Geometry: final body of the model. Coordinates: model frame, mm. A direction names the side the tool comes from. Give positions to 0.01 mm unless a question says otherwise; leave off trailing zeros. Loops run counter-clockwise (first coordinate to the right, second up) from the corner with the lowest first, then second, coordinate; pieces in that order, holes last. Notation, with made-up numbers: (12, -15) -> (63, -15) arc R19 cw to (63, 3) -> close; hole circle Ø9 at (-8, 59.5). An arc over 180 degrees is marked (long way). Answer in a Markdown table with one row per item. Add a question column.
1) Section query D-D (x = 2). Return the cut outline in (y, z), plus the area to 3 significant figures.
2) Section query A-A (z = -4.38). Return the cut outline in (x, y).
3) Section query B-B (y = 2.4). Return the cut outline in (x, z), plus the area to 3 significant figures.
4) Draft query along Z for faces 1 (the flat face through (4.52, 1.48, -21.69)), 2 (the flat face through (5, 3, -12)), 3 (the cylindrical face through (3.79, 1.48, -4.05)). Return one class per face: +Z half, -Z half, draft (parallel to the pull), parting line (faces both ways), or undercut.
5) Section query C-C (z = -21). Return the cut outline in (x, y).
6) Access query for faces 4 (the flat face through (6.006, 1.479, -21.651)), 5 (the flat face through (9.254, 1, -11)). Directions: +Z, -Z, +X, -X, +Y, -Y. A direction counts if a zero-diameter tool reaches every point of the face in a straight line with its end or side. Return the directions, or none.
7) First-contact query: P1, Ø2.5, axis at x = 5.25, z = -14.38, coming from the -Y side. Flat tip, straight axial feed; report the tip coordinate or a pass-through.
8) Line query: line 1 (Z direction, x = 5.25, y = 2.65); line 2 (X direction, y = 2.05, z = -14.38); line 3 (Z direction, x = 5.75, y = 2.4). Output: solid intervals per line, ascending. Write a range as from..to.
```python
from build123d import *

# Parameters (mm, degrees)
BOSS_EXTRUDE3_DEPTH      = 3
M3_CLEARANCE_HOLE1_D     = 3
M3_CLEARANCE_HOLE1_DEPTH = 10
M3_CLEARANCE_HOLE1_TIP   = 0.901290929
SKETCH5_W                = 0.5
SKETCH5_H                = 21.724414851
CUT_EXTRUDE1_DEPTH       = 10
SKETCH6_W                = 8
SKETCH6_H                = 3
CUT_EXTRUDE2_DEPTH       = 1.38


with BuildPart() as part:
    # Sketch1 → Boss-Extrude3 (new body)
    with BuildSketch(Plane(origin=(0, 0, 0), x_dir=(1, 0, 0), z_dir=(0, 1, 0))):
        Polygon((5.303721661, 23.00020151), (5.253721661, 23.00020151), (5.253721661, 0), (9.753721661, 0), (9.753721661, 21.724414851), (9.35, 21.724414851), (6.6889675, 20.339169011), align=None)
        Polygon((3.818475821, 20.339169011), (1.157443322, 21.724414851), (0.753721661, 21.724414851), (0.753721661, 0), (5.253721661, 0), (5.253721661, 23.00020151), (5.203721661, 23.00020151), align=None)
    extrude(amount=BOSS_EXTRUDE3_DEPTH)

    # M3 Clearance Hole1
    with Locations(Plane(origin=(5.253721661, 3, -14.38), x_dir=(0, 0, 1), z_dir=(0, 1, 0))):
        with Locations((0, 0), (10, 0)):
            Hole(M3_CLEARANCE_HOLE1_D / 2, depth=M3_CLEARANCE_HOLE1_DEPTH)
            with Locations((0, 0, -(M3_CLEARANCE_HOLE1_DEPTH + M3_CLEARANCE_HOLE1_TIP / 2))):  # 118° drill point
                Cone(0, M3_CLEARANCE_HOLE1_D / 2, M3_CLEARANCE_HOLE1_TIP, mode=Mode.SUBTRACT)

    # Sketch5 → Cut-Extrude1 (cut)
    with BuildSketch(Plane(origin=(0, 0, 0), x_dir=(-1, 0, 0), z_dir=(0, -1, 0))):
        with Locations((-1.003721661, 10.862207426)):
            Rectangle(SKETCH5_W, SKETCH5_H)
        with Locations((-9.503721661, 10.862207426)):
            Rectangle(SKETCH5_W, SKETCH5_H)
    extrude(amount=-CUT_EXTRUDE1_DEPTH, mode=Mode.SUBTRACT)

    # Sketch6 → Cut-Extrude2 (cut)
    with BuildSketch(Plane.XY):
        with Locations((5.253721661, 1.5)):
            Rectangle(SKETCH6_W, SKETCH6_H)
    extrude(amount=-CUT_EXTRUDE2_DEPTH, mode=Mode.SUBTRACT)


solid = part.part
```
Evaluation:
| question | item | result |
|---|---|---|
| 1 | outline | (0, -21.29) -> (3, -21.29) -> (3, -1.38) -> (0, -1.38) -> close |
| 1 | area | 59.7 mm² |
| 2 | outline | (1.25, 0) -> (3.75, 0) -> (3.75, 3) -> (1.25, 3) -> close; (6.75, 0) -> (9.25, 0) -> (9.25, 3) -> (6.75, 3) -> close |
| 3 | outline | (1.25, -21.67) -> (3.82, -20.34) -> (5.2, -23) -> (5.3, -23) -> (6.69, -20.34) -> (9.25, -21.67) -> (9.25, -1.38) -> (1.25, -1.38) -> close; hole circle Ø3 at (5.25, -14.38); hole circle Ø3 at (5.25, -4.38) |
| 3 | area | 145 mm² |
| 4 | face 1 | -Z half |
| 4 | face 2 | draft |
| 4 | face 3 | undercut |
| 5 | outline | (1.25, 0) -> (2.55, 0) -> (2.55, 3) -> (1.25, 3) -> close; (4.16, 0) -> (6.34, 0) -> (6.34, 3) -> (4.16, 3) -> close; (7.96, 0) -> (9.25, 0) -> (9.25, 3) -> (7.96, 3) -> close |
| 6 | face 4 | -Z, +Y, -Y |
| 6 | face 5 | +Z, -Z, +X, +Y, -Y |
| 7 | P1 | through |
| 8 | line 1 | -23..-15.88, -12.88..-5.88, -2.88..-1.38 |
| 8 | line 2 | 1.25..3.75, 6.75..9.25 |
| 8 | line 3 | -22.14..-15.8, -12.96..-5.8, -2.96..-1.38 |
